from build123d import *

# Parameters (mm, degrees)
BOSS_EXTRUDE1_DEPTH = 20
SKETCH2_W           = 15
SKETCH2_H           = 10
BOSS_EXTRUDE3_DEPTH = 40
BOSS_EXTRUDE5_DEPTH = 40
SKETCH6_W           = 30
SKETCH6_H           = 15
CUT_EXTRUDE2_DEPTH  = 40
SKETCH8_W           = 0.49
SKETCH8_H           = 15
CUT_EXTRUDE4_DEPTH  = 40


with BuildPart() as part:
    # Sketch1 → Boss-Extrude1 (new body)
    with BuildSketch(Plane.XY):
        Polygon((26.1619919, -97.696960071), (26.1619919, -67.696960071), (1.1619919, -67.696960071), (1.1619919, -97.696960071), (-6.3380081, -97.696960071), (-21.3380081, -50), (-21.3380081, 0), (48.6619919, 0), (48.6619919, -50), (33.6619919, -97.696960071), align=None)
    extrude(amount=BOSS_EXTRUDE1_DEPTH)

    # Sketch2 → Boss-Extrude3 (add)
    with BuildSketch(Plane.XY):
        with Locations((41.1619919, -5)):
            Rectangle(SKETCH2_W, SKETCH2_H)
        with Locations((-13.8380081, -5)):
            Rectangle(SKETCH2_W, SKETCH2_H)
    extrude(amount=BOSS_EXTRUDE3_DEPTH)

    # Sketch4 → Boss-Extrude5 (add)
    with BuildSketch(Plane.XY):
        Polygon((-21.3380081, -30), (48.6619919, -30), (48.6619919, -10), (28.6619919, -10), (28.6619919, -24.999154542), (13.6619919, -24.999154542), (-1.3380081, -24.999154542), (-1.3380081, -10), (-21.3380081, -10), align=None)
    extrude(amount=BOSS_EXTRUDE5_DEPTH)

    # Sketch6 → Cut-Extrude2 (cut)
    with BuildSketch(Plane.XZ.offset(30)):
        with Locations((13.172194731, 32.5)):
            Rectangle(SKETCH6_W, SKETCH6_H)
    extrude(amount=-CUT_EXTRUDE2_DEPTH, mode=Mode.SUBTRACT)

    # Sketch8 → Cut-Extrude4 (cut)
    with BuildSketch(Plane.XZ.offset(30)):
        with Locations((28.417194731, 32.5)):
            Rectangle(SKETCH8_W, SKETCH8_H)
    extrude(amount=-CUT_EXTRUDE4_DEPTH, mode=Mode.SUBTRACT)


solid = part.part
Read the model definition and answer for the solid it produces. Units are mm, in the model's axes. A direction names the side the tool comes from. Give positions to 0.01 mm unless a question says otherwise; leave off trailing zeros. Loops run counter-clockwise (first coordinate to the right, second up) from the corner with the lowest first, then second, coordinate; pieces in that order, holes last. Notation, with made-up numbers: (-32.5, 57.25) - (25.5, 57.25) arc R19 ccw to (25.5, 75.25) - close; hole circle Ø7 at (67.25, 34). An arc over 180 degrees is marked (long way). Answer as CSV lines item,"result". Start each with the question number.
1) Find section A-A (z = 32). Write down the section's boundary in (x, y), then the cut area to 3 significant figures.
2) Which of the six approach directions +Z, -Z, +X, -X, +Y, -Y give full straight-line access (tool end or side, diameter ignored) to faces 4 (the face through (14, -24.999, 22)), 5 (the face through (-1.828, -20, 32)), 6 (the face through (26.162, -83, 10))?
3) Find section B-B (x = 8). Write down the section's boundary in (y, z), then the cut area to 3 significant figures.
4) Find section C-C (z = 4). Write down the section's boundary in (x, y), then the cut area to 3 significant figures.
5) Straight lines are drawn through the part: L1, parallel to X at y = -19.5, z = 20.5; L2, parallel to X at y = -9.5, z = 20.5; L3, parallel to Y at x = 3, z = 2. For each, find the intervals that lie inside material, in ascending order. Write a range as from..to.
6) Each of these flat-tipped pins is pushed along its axis until it touches: pin 1 Ø5.5 at (x, z) = (20.5, 22.5) entering from +Y; pin 2 Ø6 at (y, z) = (-88, 6.5) entering from -X; pin 3 Ø6 at (x, z) = (8.5, 25) entering from -Y; pin 4 Ø16 at (y, z) = (-86, 6) entering from +X. Where does it stop, or does it pass through?
7) Find section D-D (y = -84.5). Write down the section's boundary in (x, z), then the cut area to 3 significant figures.
8) Determine the mould class of faces 1 (the face through (-6.338, -5, 30)), 2 (the face through (30, -97.697, 10)), 3 (the face through (41.27, -73.51, 9.86)) for opening direction X: released by +X, released by -X, zero draft, split by the parting line, or undercut.
Findings below:
1,outline,"(-21.34, -30) - (-1.83, -30) - (-1.83, -10) - (-6.34, -10) - (-6.34, 0) - (-21.34, 0) - close; (28.66, -30) - (48.66, -30) - (48.66, 0) - (33.66, 0) - (33.66, -10) - (28.66, -10) - close"
1,area,"1,090 mm^2"
2,face 4,"+Z, +Y"
2,face 5,"+Z, +Y, -Y"
2,face 6,"+Z, -Z, -Y"
3,outline,"(-67.7, 0) - (0, 0) - (0, 20) - (-25, 20) - (-25, 25) - (-30, 25) - (-30, 20) - (-67.7, 20) - close"
3,area,"1,380 mm^2"
4,outline,"(-21.34, -50) - (-6.34, -97.7) - (1.16, -97.7) - (1.16, -67.7) - (26.16, -67.7) - (26.16, -97.7) - (33.66, -97.7) - (48.66, -50) - (48.66, 0) - (-21.34, 0) - close"
4,area,"5,370 mm^2"
5,L1,"-21.34..-1.34, 28.66..48.66"
5,L2,"-21.34..-6.34, 33.66..48.66"
5,L3,"-67.7..0"
6,pin 1,"y = 0"
6,pin 2,"x = -10.33"
6,pin 3,"y = -30"
6,pin 4,"x = 39.86"
7,outline,"(-10.49, 0) - (1.16, 0) - (1.16, 20) - (-10.49, 20) - close; (26.16, 0) - (37.81, 0) - (37.81, 20) - (26.16, 20) - close"
7,area,"466 mm^2"
8,face 1,"undercut"
8,face 2,"zero draft"
8,face 3,"released by +X"
